```python
from build123d import *

# Parameters (mm, degrees)
F0_R     = 5
F1_DEPTH = 8
F2_R     = 6
F2_R_2   = 5
F3_DEPTH = 40
F4_R     = 8
F4_R_2   = 6
F5_DEPTH = 6
F7_DEPTH = 5
F8_R     = 0.7


with BuildPart() as f1:
    # F0 (on Front) → F1 (new body)
    with BuildSketch(Plane.XZ):
        Circle(F0_R)
    extrude(amount=F1_DEPTH)

    # F2 (on face) → F3 (join)
    with BuildSketch(Plane.XZ.offset(8)):
        Circle(F2_R)
        Circle(F2_R_2, mode=Mode.SUBTRACT)
        Circle(F2_R_2)
    extrude(amount=F3_DEPTH)

    # F4 (on face) → F5 (join)
    with BuildSketch(Plane.XZ.offset(48)):
        Circle(F4_R)
        Circle(F4_R_2, mode=Mode.SUBTRACT)
        Circle(F4_R_2)
    extrude(amount=F5_DEPTH)

    # F6 (on face) → F7 (cut)
    with BuildSketch(Plane.XZ.offset(54)):
        Polygon((3.2881409233, -4.4123181388), (5.4652500594, 0.6414545014), (2.1771091361, 5.0537726402), (-3.2881409233, 4.4123181388), (-5.4652500594, -0.6414545014), (-2.1771091361, -5.0537726402), align=None)
    extrude(amount=-F7_DEPTH, mode=Mode.SUBTRACT)

    # F8
    f8_edges = [f1.edges().sort_by_distance(p)[0] for p in [
        (6, -28, 0),
        (-6, -8, 0),
        (-6, -48, 0),
        (-8, -54, 0),
    ]]
    fillet(f8_edges, radius=F8_R)


solid = f1.part
```
For this review, take the finished solid that the model builds, in its own axes (mm). A direction names the side the tool comes from. Give positions to 0.01 mm unless a question says otherwise; leave off trailing zeros. Write each loop counter-clockwise with the first axis right and the second up, starting at its lowest first coordinate (ties: lowest second). Pieces come first, ordered by that corner, then holes. Notation, with made-up numbers: M 74,-26 L 92,-26 A17 cw 92,-21 Z; hole C 79.25,-11.75 d10. An arc over 180 degrees is marked long. Answer as a JSON object with one key per item and string values. Group by question number.
Item 1: Consider section A-A on z = 0. Write out the cut boundary in (x, y), plus the area to 3 significant figures.
Item 2: Consider section C-C on x = 0. Write out the cut boundary in (y, z), plus the area to 3 significant figures.
Item 3: For pin 1 Ø1.5 at (x, z) = (-5.5, 4.5) entering from +Y; pin 2 Ø5 at (x, y) = (3, -43.5) entering from +Z; pin 3 Ø5 at (x, y) = (4, -26) entering from -Z, all flat-tipped, find the tip position at first contact; note any pin that passes through.
Item 4: Tool access review of faces 1 (the cylindrical face through (-1.73, -50.61, -7.81)), 2 (the flat face through (-4.36, -51.54, 1.92)), 3 (the flat face through (-5, -48, -5)): name each direction out of +Z, -Z, +X, -X, +Y, -Y from which nothing blocks a thin tool from reaching the whole face with its end or side.
Item 5: Consider section B-B on y = -18. Write out the cut boundary in (x, z), plus the area to 3 significant figures.
Item 6: For probe 1 along X at (y, z) = (-36.5, 0.25); probe 2 along X at (y, z) = (-4.5, -4.5); probe 3 along Y at (x, z) = (1, 1.5), list the stretches that pass through material, from the lowest coordinate up. Write a range as [from, to].
Check result:
{
 "1": {"outline": "M -8,-53.3 A0.7 ccw -7.3,-54 L -5.19,-54 L -5.19,-49 L 5.19,-49 L 5.19,-54 L 7.3,-54 A0.7 ccw 8,-53.3 L 8,-48 L 6.7,-48 A0.7 cw 6,-47.3 L 6,-8.7 A0.7 ccw 5.3,-8 L 5,-8 L 5,0 L -5,0 L -5,-8 L -5.3,-8 A0.7 ccw -6,-8.7 L -6,-47.3 A0.7 cw -6.7,-48 L -8,-48 Z", "area": "604 mm^2"},
 "2": {"outline": "M -54,-7.3 A0.7 ccw -53.3,-8 L -48,-8 L -48,-6.7 A0.7 cw -47.3,-6 L -8.7,-6 A0.7 ccw -8,-5.3 L -8,-5 L 0,-5 L 0,5 L -8,5 L -8,5.3 A0.7 ccw -8.7,6 L -47.3,6 A0.7 cw -48,6.7 L -48,8 L -53.3,8 A0.7 ccw -54,7.3 L -54,4.8 L -49,4.8 L -49,-4.8 L -54,-4.8 Z", "area": "608 mm^2"},
 "3": {"pin 1": "stops at y = -47.91", "pin 2": "stops at z = 5.98", "pin 3": "stops at z = -5.81"},
 "4": {"face 1": "+Y, -Y", "face 2": "-Y", "face 3": "+Y"},
 "5": {"outline": "C 0,0 d12", "area": "113 mm^2"},
 "6": {"probe 1": "x = [-5.99, 5.99]", "probe 2": "x = [-2.18, 2.18]", "probe 3": "y = [-49, 0]"}
}
